Verification items for the finished model (mm, model axes). Face numbers are marked on the shaded views. Coordinates: 2 decimals unless noted, no trailing zeros. Loops run counter-clockwise (first coordinate to the right, second up) from the corner with the lowest first, then second, coordinate; pieces in that order, holes last.
Q1. Sectioned sample at C-C (z = -8.5). Enter the section's corners in (x, y).
Q2. Sectioned sample at A-A (x = 0). Enter the section's corners in (y, z).
Q3. Material ranges on probe 1 along Y at (x, z) = (0, 8.5); probe 2 along X at (y, z) = (24.5, -21); probe 3 along Y at (x, z) = (-29, 5.5), recorded low to high.
Q4. Go/stop test with flat-tipped pins: P1, Ø3, axis at x = -9, z = -15, coming from the -Y side; P2, Ø1.5, axis at x = 7.5, z = -14, coming from the +Y side; P3, Ø3, axis at x = -14, z = 23, coming from the -Y side. Record where each tip stops, or that it passes through.
Q5. Mould release check, pull along Y, two halves, no side actions. Record for the marked faces 1, 2 and 3: +Y half, -Y half, draft (parallel to the pull), parting line (faces both ways), or undercut.
```python
from build123d import *

# Parameters (mm, degrees)
SKETCH_1_R        = 57.5
SKETCH_1_R_2      = 42.5
EXTRUDE_317_DEPTH = 29
FILLET_1_R        = 4


with BuildPart() as part:
    # Эскиз1 → Extrude 317 (new, symmetric)
    with BuildSketch(Plane.XY):
        with Locations(Location((0, 0, 0), (0, 0, 180))):
            Circle(SKETCH_1_R)
        with Locations(Location((0, 0, 0), (0, 0, 180))):
            Circle(SKETCH_1_R_2, mode=Mode.SUBTRACT)
    extrude(amount=EXTRUDE_317_DEPTH, both=True)

    # Скругление1
    fillet_1_edges = [part.edges().sort_by_distance(p)[0] for p in [
        (57.5, 0, -29),
        (57.5, 0, 29),
        (42.5, 0, -29),
        (42.5, 0, 29),
    ]]
    fillet(fillet_1_edges, radius=FILLET_1_R)


solid = part.part
```
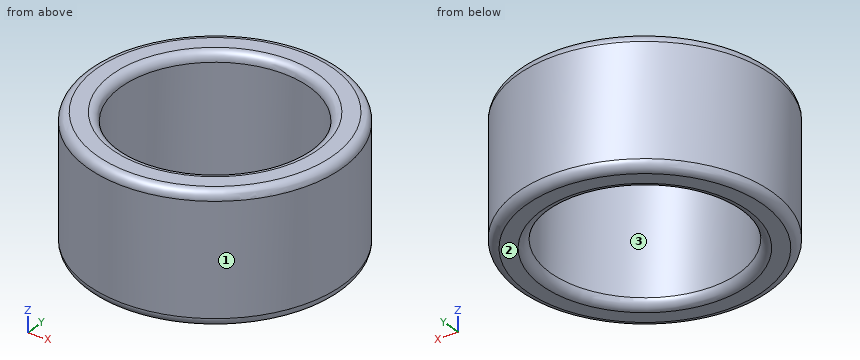
Geometry check:
1. outline: circle Ø115 at (0, 0); hole circle Ø85 at (0, 0)
2. outline: (-57.5, -25) arc R4 ccw to (-53.5, -29) - (-46.5, -29) arc R4 ccw to (-42.5, -25) - (-42.5, 25) arc R4 ccw to (-46.5, 29) - (-53.5, 29) arc R4 ccw to (-57.5, 25) - close; (42.5, -25) arc R4 ccw to (46.5, -29) - (53.5, -29) arc R4 ccw to (57.5, -25) - (57.5, 25) arc R4 ccw to (53.5, 29) - (46.5, 29) arc R4 ccw to (42.5, 25) - close
3. probe 1: y = -57.5 to -42.5, 42.5 to 57.5
3. probe 2: x = -52.02 to -34.73, 34.73 to 52.02
3. probe 3: y = -49.65 to -31.07, 31.07 to 49.65
4. P1: stops at y = -57.01
4. P2: stops at y = 57.1
4. P3: stops at y = -56.12
5. face 1: parting line
5. face 2: draft
5. face 3: undercut
